from build123d import *

# Parameters (mm, degrees)
SKETCH_2_W    = 5.6
SKETCH_2_H    = 7.57604586
SCALE_1_SCALE = 2.7
SCALE_2_SCALE = 0.72


with BuildPart() as part:
    # Sketch 1 → 旋转2 (revolve)
    with BuildSketch(Plane.XY):
        with BuildLine():
            Line((0, 4.32), (0, -4.32))
            ThreePointArc((0, -4.32), (4.32, 0), (0, 4.32))
        make_face()
    revolve(axis=Axis((0, 0, 0), (0, 1, 0)))

    # 草图2 → 旋转3 (revolve)
    with BuildSketch(Plane.XY, mode=Mode.PRIVATE) as revolve_3_sk:
        with Locations((2.8, -2.26802293)):
            Rectangle(SKETCH_2_W, SKETCH_2_H)
    revolve(revolve_3_sk.sketch.rotate(Axis((0, -6.05604586, 0), (0, 1, 0)), 180), axis=Axis((0, -6.05604586, 0), (0, 1, 0)))


with BuildPart() as part_1:
    # Масштаб1: scaled about (0, -1.786959448, 0)
    add(part.part.scale(SCALE_1_SCALE).moved(Location((0, 3.037831062, 0))))


with BuildPart() as part_2:
    # Масштаб2: scaled about (0, -1.786959449, 0)
    add(part_1.part.scale(SCALE_2_SCALE).moved(Location((0, -0.500348646, 0))))


solid = part_2.part
Design review of the part built by this model. Coordinates are the model's own, in mm. A direction names the side the tool comes from. Give positions to 0.01 mm unless a question says otherwise; leave off trailing zeros. Loops run counter-clockwise (first coordinate to the right, second up) from the corner with the lowest first, then second, coordinate; pieces in that order, holes last. Notation, with made-up numbers: M 18,19.25 L 53,19.25 A20 ccw 53,25.25 Z; hole C 29.25,-9.75 d9. An arc over 180 degrees is marked long. One line per question, with ' | ' between items. Start each with the question number.
1. Add section D-D (y = 8). Write out the cut boundary in (x, z).
2. Add section C-C (x = -1). Write out the cut boundary in (y, z).
3. Insertion check: P1, Ø4, axis at x = 8.5, z = -8.5, coming from the +Y side; P2, Ø2, axis at y = 1.5, z = -4, coming from the +X side; P3, Ø1.5, axis at x = 3.5, z = -2, coming from the +Y side. Each pin has a flat end and moves straight along its axis. Give the tip position at first contact, or say it passes through.
4. For faces 1 (the face through (-10.384, -2.619, 3.27)), 2 (the face through (6, 4.642, 6)), list the 3-axis set-ups (+Z, -Z, +X, -X, +Y, -Y) from which the entire face can be reached by the end or side of a thin tool; tool diameter is ignored.
5. Add section B-B (y = -2.25). Write out the cut boundary in (x, z), plus the area to 3 significant figures.
6. Add section A-A (z = 0). Write out the cut boundary in (x, y), plus the area to 3 significant figures.
7. To check wall thickness, follow L1, parallel to Y at x = 4.75, z = -7.5; L2, parallel to Z at x = -6, y = -4.5; L3, parallel to Y at x = -5.75, z = -1.25. State the ranges of each line that lie inside material, in increasing order.
Worked out:
1) outline: C 0,0 d11.08
2) outline: M -10.09,-10.84 L 4.64,-10.84 L 4.64,-7.8 A8.34 ccw 4.64,7.8 L 4.64,10.84 L -10.09,10.84 Z
3) P1: stops at y = 4.64 | P2: stops at x = 10.46 | P3: stops at y = 9.42
4) face 1: +Y, -Y | face 2: +Y
5) outline: C 0,0 d21.77 | area: 372 mm²
6) outline: M -10.89,-10.09 L 10.89,-10.09 L 10.89,4.64 L 7.86,4.64 A8.4 ccw -7.86,4.64 L -10.89,4.64 Z | area: 383 mm²
7) L1: y = -10.09 to 4.64 | L2: z = -9.08 to 9.08 | L3: y = -10.09 to 7.68
